Source: CAD feature listing. Evaluate the final solid. Frame: model axes, mm. Round coordinates to 2 decimals unless told otherwise and drop trailing zeros. Answer in a Markdown table with one row per item. Add a question column.
Item 1: Cut plane A-A on z = -849. Give the number of separate pieces and of enclosed holes in the cut face, and give its area (3 significant figures).
Item 2: Contact query for flat-ended pins moving along their axis: pin 1 (1 mm diameter, centred on x = -25, z = -635, fed in from -Y); pin 2 (2.5 mm diameter, centred on y = 10, z = -512, fed in from -X); pin 3 (1.8 mm diameter, centred on x = -46.5, z = -403, fed in from +Y). Output: stop coordinate, or through.
Item 3: Material intervals for probe 1 along Y at (x, z) = (-44.5, -345); probe 2 along Y at (x, z) = (-26, -887); probe 3 along X at (y, z) = (72, -358.5), sorted ascending.
from build123d import *

# Parameters (mm, degrees)
ESQUISSE1_R        = 4
BOSS_EXTRU_1_DEPTH = 998


with BuildPart() as part:
    # Esquisse1 → Boss.-Extru.1 (new body)
    with BuildSketch(Plane(origin=(0, 0, -1000), x_dir=(-1, 0, 0), z_dir=(0, 0, -1))):
        with BuildLine():
            Line((42.288948628, 57.315448094), (48.288948628, 57.315448094))
            Line((48.288948628, 57.315448094), (48.288948628, 72.815448094))
            ThreePointArc((48.288948628, 72.815448094), (47.410268972, 74.936768437), (45.288948628, 75.815448094))
            Line((45.288948628, 75.815448094), (29.788948628, 75.815448094))
            Line((29.788948628, 75.815448094), (29.788948628, 69.815448094))
            Line((29.788948628, 69.815448094), (21.788948628, 69.815448094))
            Line((21.788948628, 69.815448094), (21.788948628, 75.815448094))
            Line((21.788948628, 75.815448094), (6.288948628, 75.815448094))
            ThreePointArc((6.288948628, 75.815448094), (4.167628284, 74.936768437), (3.288948628, 72.815448094))
            Line((3.288948628, 72.815448094), (3.288948628, 57.315448094))
            Line((3.288948628, 57.315448094), (9.288948628, 57.315448094))
            Line((9.288948628, 57.315448094), (9.288948628, 49.315448094))
            Line((9.288948628, 49.315448094), (3.288948628, 49.315448094))
            Line((3.288948628, 49.315448094), (3.288948628, 12.315448094))
            Line((3.288948628, 12.315448094), (9.288948628, 12.315448094))
            Line((9.288948628, 12.315448094), (9.288948628, 4.315448094))
            Line((9.288948628, 4.315448094), (3.288948628, 4.315448094))
            Line((3.288948628, 4.315448094), (3.288948628, -11.184551906))
            ThreePointArc((3.288948628, -11.184551906), (4.167628284, -13.30587225), (6.288948628, -14.184551906))
            Line((6.288948628, -14.184551906), (21.788948628, -14.184551906))
            Line((21.788948628, -14.184551906), (21.788948628, -8.184551906))
            Line((21.788948628, -8.184551906), (29.788948628, -8.184551906))
            Line((29.788948628, -8.184551906), (29.788948628, -14.184551906))
            Line((29.788948628, -14.184551906), (45.288948628, -14.184551906))
            ThreePointArc((45.288948628, -14.184551906), (47.410268972, -13.30587225), (48.288948628, -11.184551906))
            Line((48.288948628, -11.184551906), (48.288948628, 4.315448094))
            Line((48.288948628, 4.315448094), (42.288948628, 4.315448094))
            Line((42.288948628, 4.315448094), (42.288948628, 12.315448094))
            Line((42.288948628, 12.315448094), (48.288948628, 12.315448094))
            Line((48.288948628, 12.315448094), (48.288948628, 49.315448094))
            Line((48.288948628, 49.315448094), (42.288948628, 49.315448094))
            Line((42.288948628, 49.315448094), (42.288948628, 57.315448094))
        make_face()
        with Locations((25.788948628, 53.315448094)):
            Circle(ESQUISSE1_R, mode=Mode.SUBTRACT)
        with Locations((25.788948628, 8.315448094)):
            Circle(ESQUISSE1_R, mode=Mode.SUBTRACT)
    extrude(amount=-BOSS_EXTRU_1_DEPTH)


solid = part.part
Results below:
| question | item | result |
|---|---|---|
| 1 | separate pieces | 1 |
| 1 | enclosed holes | 2 |
| 1 | area | 3,650 mm2 |
| 2 | pin 1 | y = -8.18 |
| 2 | pin 2 | x = -42.29 |
| 2 | pin 3 | y = 75.8 |
| 3 | probe 1 | -14.18 to 4.32, 12.32 to 49.32, 57.32 to 75.82 |
| 3 | probe 2 | -8.18 to 4.32, 12.31 to 49.32, 57.31 to 69.82 |
| 3 | probe 3 | -48.29 to -29.79, -21.79 to -3.29 |
